For this review, take the finished solid that the model builds, in its own axes (mm). A direction names the side the tool comes from. Give positions to 0.01 mm unless a question says otherwise; leave off trailing zeros. Loops run counter-clockwise (first coordinate to the right, second up) from the corner with the lowest first, then second, coordinate; pieces in that order, holes last. Notation, with made-up numbers: (39.25, 37.5) -> (50.25, 37.5) arc R31 cw to (50.25, 63.5) -> close; hole circle Ø10 at (77.5, 62). An arc over 180 degrees is marked (long way). Answer as CSV lines item,"result". Start each with the question number.
Item 1: For L1, parallel to X at y = -56, z = 49; L2, parallel to Y at x = -90.5, z = 55.5; L3, parallel to Y at x = -2, z = 34, list the stretches that pass through material, from the lowest coordinate up. Write a range as from..to.
Item 2: Machinability: for faces 1 (the face through (-75.85, 6.13, 33.76)), 2 (the face through (1.38, -6.2, 32.19)), which of the approach directions +Z, -Z, +X, -X, +Y, -Y give a long, thin tool a straight path to every point of the face, cutting with its end or side? Answer none if there is none.
Item 3: Add section D-D on x = -119.5. State the section outline as (y, z) points (3 decimals).
Item 4: Add section B-B on x = -84. State the section outline as (y, z) points (3 decimals), plus the area to 3 significant figures.
Item 5: The part is to be moulded in two halves that separate along X. For faces 3 (the face through (2, -35, 0)), 4 (the face through (36.479, -164.273, 31.306)), 5 (the face through (-46.667, -61.701, 33.76)), say which applies: +X half, -X half, draft (parallel to the pull), parting line (faces both ways), or undercut.
Item 6: Add section C-C on y = -87. State the section outline as (x, z) points (3 decimals).
Item 7: Clearance check with flat-ended pins moving along their axes: P1, Ø6, axis at x = 28.5, z = 53.5, coming from the -Y side; P2, Ø11.5, axis at x = 0, y = 0, coming from the -Z side; P3, Ø1, axis at x = -39.5, z = 45, coming from the -Y side; P4, Ø12, axis at y = 61, z = 52, coming from the +X side. State where each tip first meets the part, or that it passes through.
Item 8: Add section A-A on z = 34. State how many separate pieces and enclosed holes the cut face has, plus the area to 3 significant figures.
```python
from build123d import *

# Parameters (mm, degrees)
F4_DEPTH        = 60.325
F4_COPIES_COUNT = 6


# Not quite as in the source:
# - a pattern or mirror of a feature is missing from the dataset's text; its kind, count and spacing are read off the source's solid


with BuildPart() as f2:
    # F0 (on Front) → F2 (revolve)
    with BuildSketch(Plane.XZ):
        Polygon((-9.525, 0), (-6.35, 0), (-6.35, 63.5), (-9.525, 63.5), (-9.525, 38.1), (-9.525, 3.175), (-18.9311246582, 3.175), (-139.6226100799, 3.175), (-165.1, 3.175), (-165.1, 38.1), (-165.1, 63.5), (-168.275, 63.5), (-168.275, 0), (-165.1, 0), (-139.7, 0), (-19.05, 0), align=None)
    revolve(axis=Axis((0, 0, 2.6372056454), (0, 0, -1)))

    # F3 (on face) → F4 (join, through all)
    with BuildSketch(Plane.XY.offset(63.5)):
        with BuildLine():
            Line((-92.1809510877, -117.3489364313), (7.0995158286, -6.35))
            ThreePointArc((7.0995158286, -6.35), (3.8885649667, -8.6950956004), (0, -9.525))
            Line((0, -9.525), (-94.6602110475, -115.3583333333))
            ThreePointArc((-94.6602110475, -115.3583333333), (-93.4258828815, -116.3602381951), (-92.1809510877, -117.3489364313))
        make_face()
    f4 = extrude(amount=-F4_DEPTH)

    # F4_copies: F4 ×6 about axis
    f4_copies_axis = Axis((0, 0, 0), (0, 0, 1))
    for i in range(1, F4_COPIES_COUNT):
        add(f4.rotate(f4_copies_axis, i * 360 / F4_COPIES_COUNT))


solid = f2.part
```
Computed values:
1,L1,"-158.68..-155.31, -41.57..-37.31, 25.08..28.43, 155.31..158.68"
1,L2,"-141.87..-138.09, -115.47..-110.71, 9.19..12.44, 138.09..141.87"
1,L3,"-168.26..-165.09, -16.52..-11.76, -9.31..-6.03, 6.03..12.05, 165.09..168.26"
2,face 1,"+Z"
2,face 2,"+Z, -Z"
3,outline,"(-118.475, 0) -> (118.475, 0) -> (118.475, 63.5) -> (113.92, 63.5) -> (113.92, 3.175) -> (18.5, 3.175) -> (18.5, 63.5) -> (15.256, 63.5) -> (15.256, 3.175) -> (-113.92, 3.175) -> (-113.92, 63.5) -> (-118.475, 63.5) -> close"
4,outline,"(-145.81, 0) -> (145.81, 0) -> (145.81, 63.5) -> (142.134, 63.5) -> (142.134, 3.175) -> (11.077, 3.175) -> (11.077, 63.5) -> (7.833, 63.5) -> (7.833, 3.175) -> (-103.44, 3.175) -> (-103.44, 63.5) -> (-108.202, 63.5) -> (-108.202, 3.175) -> (-142.134, 3.175) -> (-142.134, 63.5) -> (-145.81, 63.5) -> close"
4,area,"1,850 mm²"
5,face 3,"draft"
5,face 4,"parting line"
5,face 5,"undercut"
6,outline,"(-144.04, 0) -> (144.04, 0) -> (144.04, 63.5) -> (140.318, 63.5) -> (140.318, 3.175) -> (38.613, 3.175) -> (38.613, 63.5) -> (35.271, 63.5) -> (35.271, 3.175) -> (-65.036, 3.175) -> (-65.036, 63.5) -> (-69.296, 63.5) -> (-69.296, 3.175) -> (-140.318, 3.175) -> (-140.318, 63.5) -> (-144.04, 63.5) -> close"
7,P1,"y = -166.33"
7,P2,"through"
7,P3,"y = -163.69"
7,P4,"x = 159.03"
8,separate pieces,"2"
8,enclosed holes,"2"
8,area,"6,230 mm²"
